Could you check a few things on this model? Use its own coordinates, in mm. A direction names the side the tool comes from. Coordinates: 2 decimals unless noted, no trailing zeros. Write each loop counter-clockwise with the first axis right and the second up, starting at its lowest first coordinate (ties: lowest second). Pieces come first, ordered by that corner, then holes.
Autodesk Inventor part; units mm, degrees
ref_plane "YZ Plane" through (0, 0, 0) normal (1, 0, 0) x (0, 1, 0)
ref_plane "XZ Plane" through (0, 0, 0) normal (0, 1, 0) x (-1, 0, 0)
ref_plane "XY Plane" through (0, 0, 0) normal (0, 0, 1) x (1, 0, 0)
sketch "Skizze1" plane through (0, 0, 0) normal (0, 0, 1) x (1, 0, 0)
  circle A0 centre (0, 0) radius 34.775
  dimension "d0" = 69.55
extrude "Extrusion1" add sketch "Skizze1" along normal blind 5
sketch "Skizze2" plane through (0, 0, 5) normal (0, 0, 1) x (1, 0, 0)
  circle A0 centre (0, 0) radius 32.54
  dimension "d3" = 65.08
extrude "Extrusion2" cut sketch "Skizze2" against normal blind 3
sketch "Skizze3" plane through (0, 0, 0) normal (0, 0, -1) x (-1, 0, 0)
  circle A0 centre (0, 0) radius 7.25
  dimension "d6" = 14.5
extrude "Extrusion3" cut sketch "Skizze3" against normal through all
sketch "Skizze4" plane through (0, 0, 5) normal (0, 0, 1) x (1, 0, 0)
  line L0 (-8, -26.775) -> (8, -26.775)
  line L1 (8, -26.775) -> (8, -42.775)
  line L2 (8, -42.775) -> (-8, -42.775)
  line L3 (-8, -42.775) -> (-8, -26.775)
  circle A0 centre (0, 0) radius 34.775
  line L4 (-8, -26.775) -> (8, -42.775) construction
  line L5 (8, -26.775) -> (-8, -42.775) construction
  point P0 (0, -34.775)
  dimension "d9" = 16
  dimension "d10" = 16
extrude "Extrusion4" cut sketch "Skizze4" against normal up to surface (3 mm away) contours L0 L1 A0 L3 | A0 L1 L2 L3 picked at (0.896, -29.407)
properties part number "2024_08_28_Holder_disk_NS14"
Item 1: I want a section at B-B, the plane y = 0. List the corners of the cut face in (x, z) for me (3 decimals).
Item 2: I want a section at A-A, the plane x = 0. List the corners of the cut face in (y, z) for me (3 decimals).
Item 3: Which directions (+Z, -Z, +X, -X, +Y, -Y) give clear straight access to the entire face, cutting with the end or side of a thin tool? Please do faces 4 (the flat face through (10.1, 31.1, 5)), 5 (the flat face through (8, -33, 4)), 6 (the cylindrical face through (1.318, 32.513, 3.521)).
Item 4: I want a section at C-C, the plane y = 25.5. List the corners of the cut face in (x, z) for me, then the cut area to 3 significant figures.
Item 5: Will these pins go through, and if not, where does the flat tip stop? pin 1 Ø1 at (y, z) = (7, 1) entering from +X; pin 2 Ø2.5 at (y, z) = (-33, 3.5) entering from -X; pin 3 Ø23 at (x, y) = (0, 0) entering from +Z; pin 4 Ø6 at (x, y) = (24, 18) entering from +Z.
Item 6: If we mould it in two halves opening along X, with no side actions, what happens to faces 1 (the cylindrical face through (-7.539, 33.948, 2.465)), 2 (the flat face through (0, 8, 0)), 3 (the cylindrical face through (-3.35, -6.43, 0.99))? For each: released by +X, released by -X, zero draft, split by the parting line, or undercut.
Item 7: If I drill on line 1 along Y through (x, z) = (0.5, 1.3); line 2 along Z through (x, y) = (15, -14); line 3 along X through (y, z) = (0, 4) (3 decimals), over which ranges is the centre line in solid material (lowest first)?
Taken from the geometry:
1. outline: (-34.775, 0) - (-7.25, 0) - (-7.25, 2) - (-32.54, 2) - (-32.54, 5) - (-34.775, 5) - close; (7.25, 0) - (34.775, 0) - (34.775, 5) - (32.54, 5) - (32.54, 2) - (7.25, 2) - close
2. outline: (-34.775, 0) - (-7.25, 0) - (-7.25, 2) - (-34.775, 2) - close; (7.25, 0) - (34.775, 0) - (34.775, 5) - (32.54, 5) - (32.54, 2) - (7.25, 2) - close
3. face 4: +Z, +X, -X, +Y, -Y
3. face 5: +Z, -Y
3. face 6: +Z
4. outline: (-23.64, 0) - (23.64, 0) - (23.64, 5) - (20.21, 5) - (20.21, 2) - (-20.21, 2) - (-20.21, 5) - (-23.64, 5) - close
4. area: 115 mm2
5. pin 1: stops at x = 34.16
5. pin 2: stops at x = -14.19
5. pin 3: stops at z = 2
5. pin 4: stops at z = 5
6. face 1: split by the parting line
6. face 2: zero draft
6. face 3: undercut
7. line 1: y = -34.77 to -7.23, 7.23 to 34.77
7. line 2: z = 0 to 2
7. line 3: x = -34.775 to -32.54, 32.54 to 34.775
